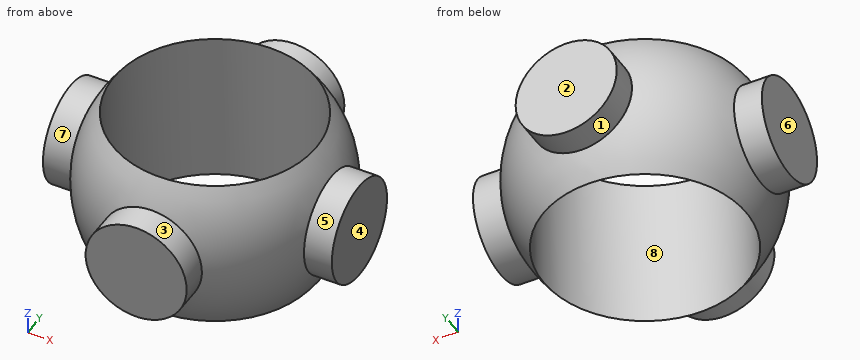
from build123d import *

# Parameters (mm, degrees)
F0_R     = 2.2225
F3_DEPTH = 6.35
F1_R     = 2.2225
F4_DEPTH = 6.35
F6_R     = 4.445
F7_DEPTH = 12.7


with BuildPart() as f3:
    # F0 (on Right) → F3 (new body, symmetric)
    with BuildSketch(Plane.YZ):
        Circle(F0_R)
    extrude(amount=F3_DEPTH, both=True)

    # F1 (on Front) → F4 (join, symmetric)
    with BuildSketch(Plane.XZ):
        Circle(F1_R)
    extrude(amount=F4_DEPTH, both=True)

    # F2 (on Right) → F5 (revolve)
    with BuildSketch(Plane.YZ):
        with BuildLine():
            Line((0, 5.588), (0, -5.588))
            ThreePointArc((0, -5.588), (5.588, 0), (0, 5.588))
        make_face()
    revolve(axis=Axis((0, 0, -0.972137), (0, 0, -1)))

    # F6 (on Top) → F7 (cut, symmetric)
    with BuildSketch(Plane.XY):
        Circle(F6_R)
    extrude(amount=F7_DEPTH, both=True, mode=Mode.SUBTRACT)


solid = f3.part
Design review of the part built by this model. Coordinates are the model's own, in mm. Face numbers are marked on the shaded views. A direction names the side the tool comes from. Give positions to 0.01 mm unless a question says otherwise; leave off trailing zeros. Order: outer loops, then holes, each group sorted by start corner. A loop starts at its lowest first (then second) coordinate and runs counter-clockwise, first axis right, second up. Notation, with made-up numbers: (-2.5, -11) - (42.5, -11) arc R13 cw to (42.5, -4) - close; hole circle Ø8 at (54.25, 27.25). An arc over 180 degrees is marked (long way). Write item = value, one per line. Start each with the question number.
Q1. To check wall thickness, follow L1, parallel to Y at x = 0, z = 1.5 (3 decimals); L2, parallel to X at y = -2.25, z = 2.5. State the ranges of each line that lie inside material, in increasing order. Write a range as from..to.
Q2. We need section D-D on z = 0.75. State the section outline as (x, y) points (3 decimals), plus the area to 3 significant figures.
Q3. Mouldability with a two-part tool opening along Y and no side actions: class the marked faces 6, 7 and 8 as released by +Y, released by -Y, zero draft, split by the parting line, or undercut.
Q4. Clearance check with flat-ended pins moving along their axes: pin 1 Ø1 at (x, y) = (4, 1.5) entering from -Z; pin 2 Ø3 at (y, z) = (4, 0) entering from -X. State where each tip first meets the part, or that it passes through.
Q5. Tool access review of the marked faces 1, 2, 3, 4 and 5: name each direction out of +Z, -Z, +X, -X, +Y, -Y from which nothing blocks a thin tool from reaching the whole face with its end or side.
Q6. We need section C-C on z = 2. State the section outline as (x, y) points (3 decimals), plus the area to 3 significant figures.
Working result:
q1.L1 = -6.35..-4.445, 4.445..6.35
q1.L2 = -4.46..-3.83, 3.83..4.46
q2.outline = (-6.35, -2.092) - (-5.127, -2.092) arc R5.537 ccw to (-2.092, -5.127) - (-2.092, -6.35) - (2.092, -6.35) - (2.092, -5.127) arc R5.537 ccw to (5.127, -2.092) - (6.35, -2.092) - (6.35, 2.092) - (5.127, 2.092) arc R5.537 ccw to (2.092, 5.127) - (2.092, 6.35) - (-2.092, 6.35) - (-2.092, 5.127) arc R5.537 ccw to (-5.127, 2.092) - (-6.35, 2.092) - close; hole circle Ø8.89 at (0, 0)
q2.area = 50.1 mm²
q3.face_6 = zero draft
q3.face_7 = split by the parting line
q3.face_8 = undercut
q4.pin_1 = -3.39
q4.pin_2 = -5
q5.face_1 = +Y
q5.face_2 = +Z, -Z, +X, -X, +Y
q5.face_3 = -Y
q5.face_4 = +Z, -Z, +X, +Y, -Y
q5.face_5 = +X
q6.outline = (-6.35, -0.969) - (-5.127, -0.969) arc R5.218 ccw to (-0.969, -5.127) - (-0.969, -6.35) - (0.969, -6.35) - (0.969, -5.127) arc R5.218 ccw to (5.127, -0.969) - (6.35, -0.969) - (6.35, 0.969) - (5.127, 0.969) arc R5.218 ccw to (0.969, 5.127) - (0.969, 6.35) - (-0.969, 6.35) - (-0.969, 5.127) arc R5.218 ccw to (-5.127, 0.969) - (-6.35, 0.969) - close; hole circle Ø8.89 at (0, 0)
q6.area = 32.5 mm²
